from build123d import *

# Parameters (mm, degrees)
SKETCH1_R               = 3.175
BOSS_EXTRUDE1_DEPTH     = 50.8
CHAMFER1_SIZE           = 0.508
SKETCH2_R               = 1.5875
CUT_EXTRUDE1_DEPTH      = 50.8
CUT_EXTRUDE1_DEPTH_BACK = 50.8


with BuildPart() as part:
    # Sketch1 → Boss-Extrude1 (new body)
    with BuildSketch(Plane(origin=(0, 0, 0), x_dir=(1, 0, 0), z_dir=(0, 1, 0))):
        Circle(SKETCH1_R)
    extrude(amount=BOSS_EXTRUDE1_DEPTH)

    # Chamfer1
    chamfer1_edges = [part.edges().sort_by_distance(p)[0] for p in [
        (-3.175, 0, 0),
        (-3.175, 50.8, 0),
    ]]
    chamfer(chamfer1_edges, length=CHAMFER1_SIZE)

    # Sketch2 → Cut-Extrude1 (cut, two sides)
    with BuildSketch(Plane.XY) as cut_extrude1_sk:
        with Locations((0, 46.99)):
            Circle(SKETCH2_R)
        with Locations((0, 18.4785)):
            Circle(SKETCH2_R)
    extrude(amount=CUT_EXTRUDE1_DEPTH, mode=Mode.SUBTRACT)
    extrude(cut_extrude1_sk.sketch, amount=-CUT_EXTRUDE1_DEPTH_BACK, mode=Mode.SUBTRACT)


solid = part.part
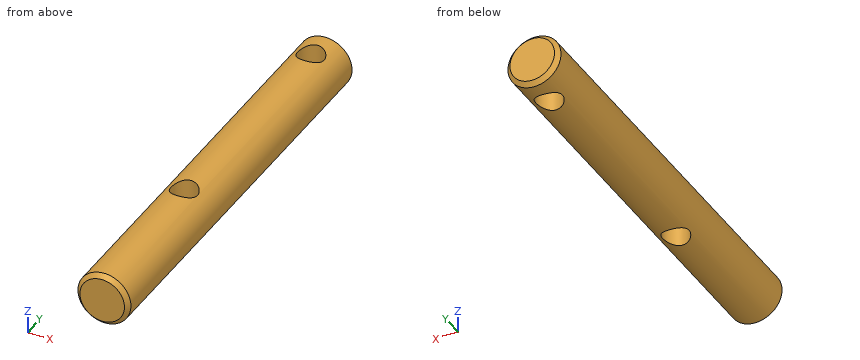
The model under review builds one solid part; all positions refer to its coordinate system, in mm. Coordinates: 2 decimals unless noted, no trailing zeros. Write each loop counter-clockwise with the first axis right and the second up, starting at its lowest first coordinate (ties: lowest second). Pieces come first, ordered by that corner, then holes. Notation, with made-up numbers: (65, 64) -> (121, 64) arc R23 cw to (121, 96) -> close; hole circle Ø4 at (-2, 13). An arc over 180 degrees is marked (long way). Answer in a Markdown table with one row per item.
1. We need section B-B, the plane z = 0. State the section outline as (x, y) points (1 decimal), and give its area (3 significant figures).
Answers below:
| item | result |
|---|---|
| outline | (-3.2, 0.5) -> (-2.7, 0) -> (2.7, 0) -> (3.2, 0.5) -> (3.2, 50.3) -> (2.7, 50.8) -> (-2.7, 50.8) -> (-3.2, 50.3) -> close; hole circle Ø3.2 at (0, 18.5); hole circle Ø3.2 at (0, 47) |
| area | 306 mm^2 |
2. We need section A-A, the plane x = 0. State the section outline as (y, z) points (1 decimal), and give its area (3 significant figures).
Answers below:
| item | result |
|---|---|
| outline | (0, -2.7) -> (0.5, -3.2) -> (16.9, -3.2) -> (16.9, 3.2) -> (0.5, 3.2) -> (0, 2.7) -> close; (20.1, -3.2) -> (45.4, -3.2) -> (45.4, 3.2) -> (20.1, 3.2) -> close; (48.6, -3.2) -> (50.3, -3.2) -> (50.8, -2.7) -> (50.8, 2.7) -> (50.3, 3.2) -> (48.6, 3.2) -> close |
| area | 282 mm^2 |
3. Clearance check with flat-ended pins moving along their axes: pin 1 Ø1.5 at (x, y) = (2.5, 44) entering from +Z; pin 2 Ø1.9 at (x, y) = (0, 46.99) entering from +Z; pin 3 Ø1 at (x, y) = (-1, 12) entering from -Z; pin 4 Ø1 at (x, z) = (-2.5, -2) entering from -Y. State where each tip first meets the part, or that it passes through.
Answers below:
| item | result |
|---|---|
| pin 1 | stops at z = 2.65 |
| pin 2 | passes through |
| pin 3 | stops at z = -3.14 |
| pin 4 | stops at y = 0.03 |
4. Wall thickness on probe 1 along Y at (x, z) = (0, -1); probe 2 along Y at (x, z) = (-0.5, 1.5); probe 3 along X at (y, z) = (46.99, -1.25): over which ranges is each line inside the solid? List them lowest first. Write a range as [from, to].
Answers below:
| item | result |
|---|---|
| probe 1 | y = [0, 16.89], [20.07, 45.4], [48.58, 50.8] |
| probe 2 | y = [0, 16.97], [19.99, 45.48], [48.5, 50.8] |
| probe 3 | x = [-2.92, -1.59], [1.59, 2.92] |
5. We need section D-D, the plane y = 8.5. State the section outline as (x, z) points (3 decimals), and give its area (3 significant figures).
Answers below:
| item | result |
|---|---|
| outline | circle Ø6.35 at (0, 0) |
| area | 31.7 mm^2 |
